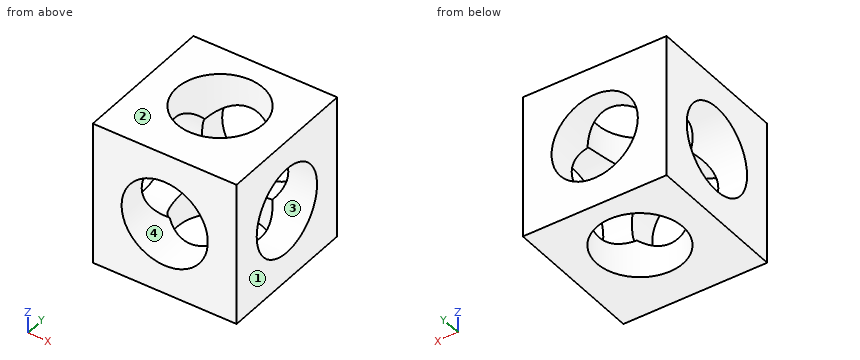
from build123d import *

# Parameters (mm, degrees)
F0_W     = 127
F0_H     = 127
F1_DEPTH = 127
F4_R     = 38.1
F5_DEPTH = 127
F3_R     = 38.1
F6_DEPTH = 127
F2_R     = 38.1
F7_DEPTH = 127


with BuildPart() as f1:
    # F0 (on Top) → F1 (new body)
    with BuildSketch(Plane.XY):
        with Locations((-63.5, 63.5)):
            Rectangle(F0_W, F0_H)
    extrude(amount=F1_DEPTH)

    # F4 (on face) → F5 (cut)
    with BuildSketch(Plane.XY.offset(127)):
        with Locations((-63.5, 69.870859)):
            Circle(F4_R)
    extrude(amount=-F5_DEPTH, mode=Mode.SUBTRACT)

    # F3 (on face) → F6 (cut)
    with BuildSketch(Plane(origin=(0, 127, 0), x_dir=(-1, 0, 0), z_dir=(0, 1, 0))):
        with Locations((63.5, 63.5)):
            Circle(F3_R)
    extrude(amount=-F6_DEPTH, mode=Mode.SUBTRACT)

    # F2 (on face) → F7 (cut)
    with BuildSketch(Plane(origin=(-127, 0, 0), x_dir=(0, -1, 0), z_dir=(-1, 0, 0))):
        with Locations((-63.5, 63.5)):
            Circle(F2_R)
    extrude(amount=-F7_DEPTH, mode=Mode.SUBTRACT)


solid = f1.part
Check sheet for the modelled part. Datum: model origin and axes. Units: mm. Face numbers are marked on the shaded views. Give positions to 0.01 mm unless a question says otherwise; leave off trailing zeros. Write each loop counter-clockwise with the first axis right and the second up, starting at its lowest first coordinate (ties: lowest second). Pieces come first, ordered by that corner, then holes. Notation, with made-up numbers: (18.25, 77) -> (56.25, 77) arc R19 ccw to (56.25, 82) -> close; hole circle Ø3 at (-15, -29.75). An arc over 180 degrees is marked (long way). One line per item, written item: value. Start each with the question number.
Item 1: Section check D-D on y = 111.5. Record the cut outline in (x, z).
Item 2: Section check B-B on z = 63.5. Record the cut outline in (x, y), then the cut area to 3 significant figures.
Item 3: Material ranges on probe 1 along Z at (x, y) = (-63, 22); probe 2 along Y at (x, z) = (-63.5, 14.5); probe 3 along X at (y, z) = (28, 34.5), recorded low to high. Write a range as from..to.
Item 4: Section check C-C on x = -21. Record the cut outline in (y, z).
Item 5: Draft check along Z on the marked faces 1, 2, 3 and 4. Enter one of: +Z half, -Z half, draft (parallel to the pull), parting line (faces both ways), or undercut.
Item 6: Section check A-A on x = -63.5. Record the cut outline in (y, z), then the cut area to 3 significant figures.
Results list:
1. outline: (-127, 0) -> (0, 0) -> (0, 127) -> (-127, 127) -> close; hole circle Ø76.2 at (-63.5, 63.5)
2. outline: (-127, 0) -> (-101.6, 0) -> (-101.6, 25.4) -> (-127, 25.4) -> close; (-127, 101.6) -> (-101.6, 101.6) -> (-101.6, 127) -> (-127, 127) -> close; (-25.4, 0) -> (0, 0) -> (0, 25.4) -> (-25.4, 25.4) -> close; (-25.4, 101.6) -> (0, 101.6) -> (0, 127) -> (-25.4, 127) -> close
2. area: 2,580 mm²
3. probe 1: 0..25.4, 101.6..127
3. probe 2: 0..31.77, 107.97..127
3. probe 3: -127..-88.21, -38.79..0
4. outline: (0, 0) -> (127, 0) -> (127, 127) -> (0, 127) -> close; hole circle Ø76.2 at (63.5, 63.5)
5. face 1: draft
5. face 2: +Z half
5. face 3: undercut
5. face 4: undercut
6. outline: (0, 0) -> (31.77, 0) -> (31.77, 25.4) -> (0, 25.4) -> close; (0, 101.6) -> (31.77, 101.6) -> (31.77, 127) -> (0, 127) -> close; (107.97, 0) -> (127, 0) -> (127, 25.4) -> (107.97, 25.4) -> close; (107.97, 101.6) -> (127, 101.6) -> (127, 127) -> (107.97, 127) -> close
6. area: 2,580 mm²
